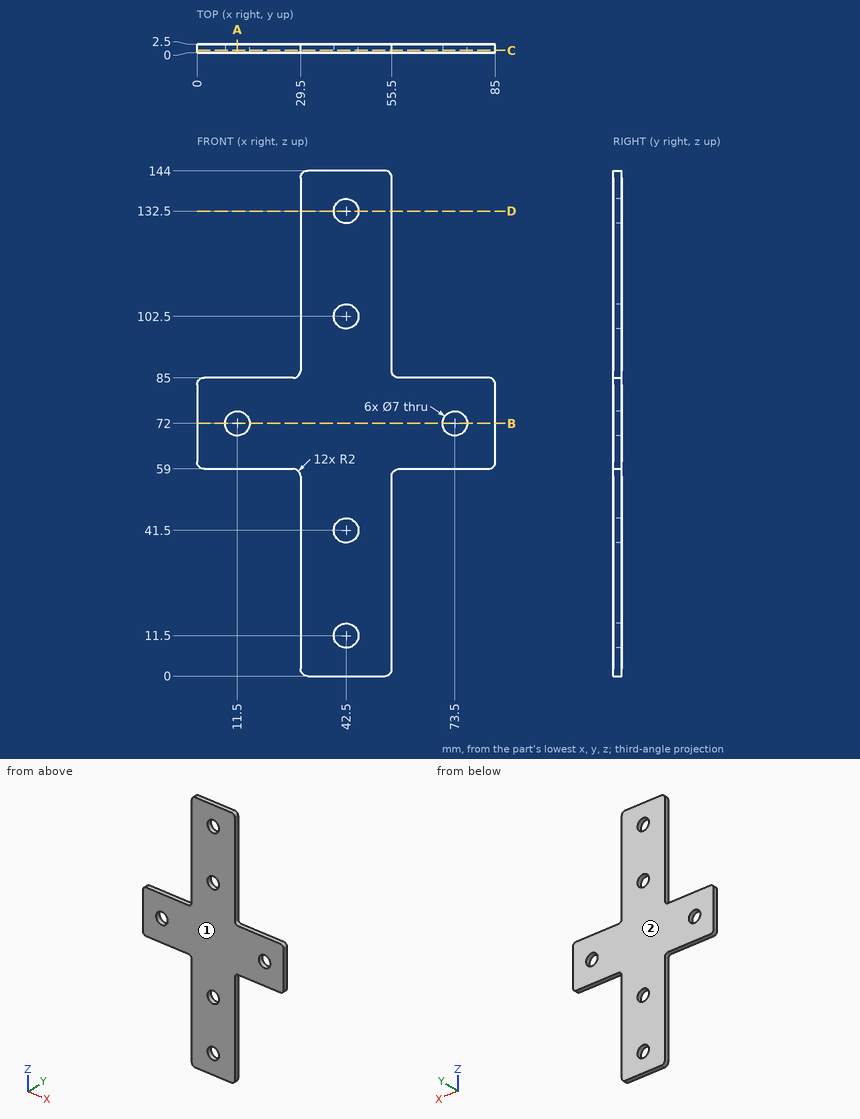
Geometry: see drawing. Coordinates: mm, zero at the bounding-box minimum. Give positions to 0.01 mm unless a question says otherwise; leave off trailing zeros. Loops run counter-clockwise (first coordinate to the right, second up) from the corner with the lowest first, then second, coordinate; pieces in that order, holes last. Notation, with made-up numbers: (-13.75, 54.5) - (9.25, 54.5) arc R35 ccw to (9.25, 93.5) - close; hole circle Ø3 at (1.5, -10). An arc over 180 degrees is marked (long way). Use CSV: the item, a comma, the result in double quotes. Start each with the question number.
1. Section B-B (z = 72). Output: boundary loops of the cut face in (x, y), then the cut area to 4 significant figures.
2. Section D-D (z = 132.5). Output: boundary loops of the cut face in (x, y), then the cut area to 3 significant figures.
3. Section C-C (y = 0.7). Count the separate pieces of the cut face and the enclosed holes in it, then the cut area to 3 significant figures.
4. Pin query (flat end, axial travel): pin 1 (6.5 mm diameter, centred on x = 42.5, z = 41.5, fed in from +Y); pin 2 (1.2 mm diameter, centred on y = 1.5, z = 116, fed in from +X); pin 3 (1.2 mm diameter, centred on x = 69.5, y = 1.5, fed in from +Z); pin 4 (1.2 mm diameter, centred on y = 1.5, z = 127.5, fed in from -X). Return the tip coordinate at first contact, or that it passes through.
5. Draft query along Y for the marked faces 1 and 2. Return one class per face: +Y half, -Y half, draft (parallel to the pull), parting line (faces both ways), or undercut.
6. Section A-A (x = 11.5). Output: boundary loops of the cut face in (y, z), then the cut area to 3 significant figures.
7. Ray query, L1, parallel to Z at x = 42.5, y = 0.9; L2, parallel to X at y = 1.5, z = 72; L3, parallel to X at y = 0.65, z = 132.5. Return the intervals inside material, ascending.
Response:
1,outline,"(0, 0) - (8, 0) - (8, 2.5) - (0, 2.5) - close; (15, 0) - (70, 0) - (70, 2.5) - (15, 2.5) - close; (77, 0) - (85, 0) - (85, 2.5) - (77, 2.5) - close"
1,area,"177.5 mm²"
2,outline,"(29.5, 0) - (39, 0) - (39, 2.5) - (29.5, 2.5) - close; (46, 0) - (55.5, 0) - (55.5, 2.5) - (46, 2.5) - close"
2,area,"47.5 mm²"
3,separate pieces,"1"
3,enclosed holes,"6"
3,area,"5,040 mm²"
4,pin 1,"through"
4,pin 2,"x = 55.5"
4,pin 3,"z = 85"
4,pin 4,"x = 29.5"
5,face 1,"-Y half"
5,face 2,"+Y half"
6,outline,"(0, 59) - (2.5, 59) - (2.5, 68.5) - (0, 68.5) - close; (0, 75.5) - (2.5, 75.5) - (2.5, 85) - (0, 85) - close"
6,area,"47.5 mm²"
7,L1,"0 to 8, 15 to 38, 45 to 99, 106 to 129, 136 to 144"
7,L2,"0 to 8, 15 to 70, 77 to 85"
7,L3,"29.5 to 39, 46 to 55.5"
